CAD build for the part. Positions are in the model's coordinates, mm. A direction names the side the tool comes from. Coordinates: 2 decimals unless noted, no trailing zeros. Loops run counter-clockwise (first coordinate to the right, second up) from the corner with the lowest first, then second, coordinate; pieces in that order, holes last. Notation, with made-up numbers: (20.25, 85) -> (36.25, 85) arc R35 cw to (36.25, 123) -> close; hole circle Ø11 at (60.25, -18.5). An arc over 180 degrees is marked (long way). Return JSON: item names as keys, results as strings. Group by question number.
(1) Mould opens along X. For faces 1 (the face through (-30.5, 0, 6)), 2 (the face through (-32.43, -0.11, 0.6)), 3 (the face through (0.42, -9.93, 0.6)) say: pulls with the +X half, pulls with the -X half, needs draft (parallel to the pull), parting line crosses it, or undercut.
(2) Saw through at B-B on z = 7.5. Write the cut outline in (x, y), then the cut area to 3 significant figures.
(3) Tool access for faces 4 (the face through (0, 8, 6)), 5 (the face through (-32.1, 9.64, 5.94)): list every direction of +Z, -Z, +X, -X, +Y, -Y with a clear straight run to the whole face (end or side of a thin tool).
(4) Flat gauge pins, fed straight in: pin 1 Ø12 at (x, y) = (2, -3) entering from +Z; pin 2 Ø1 at (x, y) = (-1, 1) entering from +Z. Where does each tip first touch, or does it go through?
(5) Saw through at C-C on y = 0. Write the cut outline in (x, z).
(6) Probe L1, parallel to Y at x = 9, z = 4; L2, parallel to X at y = -4.75, z = 9; L3, parallel to Z at x = -4, y = -5.75. List the from-to ranges inside material, lowest first.
(7) Saw through at A-A on x = -8.5. Write the cut outline in (y, z).
```python
from build123d import *

# Parameters (mm, degrees)
F1_DEPTH = 10
F2_T     = -2.5
F3_R     = 1.9452355594
F4_DEPTH = 2.501
F6_R     = 2


# Not quite as in the source:
# - a fillet or chamfer that OpenCascade refuses, or shapes differently, is made with other operations: its cross-section is extruded or revolved along the edge and cut away or added


with BuildPart() as f1:
    # F0 (on Top) → F1 (new body)
    with BuildSketch(Plane.XY):
        with BuildLine():
            Line((-30, -10.5), (30, -10.5))
            ThreePointArc((30, -10.5), (32.1213203436, -9.6213203436), (33, -7.5))
            Line((33, -7.5), (33, 7.5))
            ThreePointArc((33, 7.5), (32.1213203436, 9.6213203436), (30, 10.5))
            Line((30, 10.5), (-30, 10.5))
            ThreePointArc((-30, 10.5), (-32.1213203436, 9.6213203436), (-33, 7.5))
            Line((-33, 7.5), (-33, -7.5))
            ThreePointArc((-33, -7.5), (-32.1213203436, -9.6213203436), (-30, -10.5))
        make_face()
    extrude(amount=F1_DEPTH)

    # F2
    f2_openings = [f1.faces().sort_by_distance(p)[0] for p in [
        (0, 0, 10),
    ]]
    offset(amount=F2_T, openings=f2_openings)

    # F3 (on face) → F4 (cut, through all)
    with BuildSketch(Plane.XY.offset(2.5)):
        with Locations((-23.9163879305, 0)):
            Circle(F3_R)
        with Locations((23.9163879305, 0)):
            Circle(F3_R)
    extrude(amount=-F4_DEPTH, mode=Mode.SUBTRACT)

    # F5: chamfer of 3 on 2 edges, made by hand

    # F5_s1 → F5_t2 (revolve, cut)
    with BuildSketch(Plane.XZ):
        Polygon((28.8616234899, 0), (25.8616234899, 3), (25.8616234899, 0), align=None)
    revolve(axis=Axis((23.9163879305, 0, 0), (0, 0, 1)), mode=Mode.SUBTRACT)

    # F5_s3 → F5_t4 (revolve, cut)
    with BuildSketch(Plane.XZ):
        Polygon((-18.9711523711, 0), (-21.9711523711, 3), (-21.9711523711, 0), align=None)
    revolve(axis=Axis((-23.9163879305, 0, 0), (0, 0, 1)), mode=Mode.SUBTRACT)

    # F6
    f6_edges = [f1.edges().sort_by_distance(p)[0] for p in [
        (0, -10.5, 0),
        (-32.12132, -9.62132, 0),
        (32.12132, -9.62132, 0),
        (-33, 0, 0),
        (33, 0, 0),
        (-32.12132, 9.62132, 0),
        (32.12132, 9.62132, 0),
        (0, 10.5, 0),
        (-28.861623, 0, 0),
        (18.971152, 0, 0),
    ]]
    fillet(f6_edges, radius=F6_R)


solid = f1.part
```
Geometry results:
{
 "1": {"face 1": "undercut", "face 2": "pulls with the -X half", "face 3": "needs draft"},
 "2": {"outline": "(-33, -7.5) arc R3 ccw to (-30, -10.5) -> (30, -10.5) arc R3 ccw to (33, -7.5) -> (33, 7.5) arc R3 ccw to (30, 10.5) -> (-30, 10.5) arc R3 ccw to (-33, 7.5) -> close; hole (-30.5, -7.5) arc R0.5 ccw to (-30, -8) -> (30, -8) arc R0.5 ccw to (30.5, -7.5) -> (30.5, 7.5) arc R0.5 ccw to (30, 8) -> (-30, 8) arc R0.5 ccw to (-30.5, 7.5) -> close", "area": "402 mm²"},
 "3": {"face 4": "+Z", "face 5": "+Z, -Z, -X, +Y"},
 "4": {"pin 1": "z = 10", "pin 2": "z = 2.5"},
 "5": {"outline": "(-33, 2) arc R2 ccw to (-31, 0) -> (-29.69, 0) arc R2 ccw to (-28.28, 0.59) -> (-26.36, 2.5) -> (-30.5, 2.5) -> (-30.5, 10) -> (-33, 10) -> close; (-21.47, 2.5) -> (-19.56, 0.59) arc R2 ccw to (-18.14, 0) -> (18.14, 0) arc R2 ccw to (19.56, 0.59) -> (21.47, 2.5) -> close; (26.36, 2.5) -> (28.28, 0.59) arc R2 ccw to (29.69, 0) -> (31, 0) arc R2 ccw to (33, 2) -> (33, 10) -> (30.5, 10) -> (30.5, 2.5) -> close"},
 "6": {"L1": "-10.5 to -8, 8 to 10.5", "L2": "-33 to -30.5, 30.5 to 33", "L3": "0 to 2.5"},
 "7": {"outline": "(-10.5, 2) arc R2 ccw to (-8.5, 0) -> (8.5, 0) arc R2 ccw to (10.5, 2) -> (10.5, 10) -> (8, 10) -> (8, 2.5) -> (-8, 2.5) -> (-8, 10) -> (-10.5, 10) -> close"}
}
